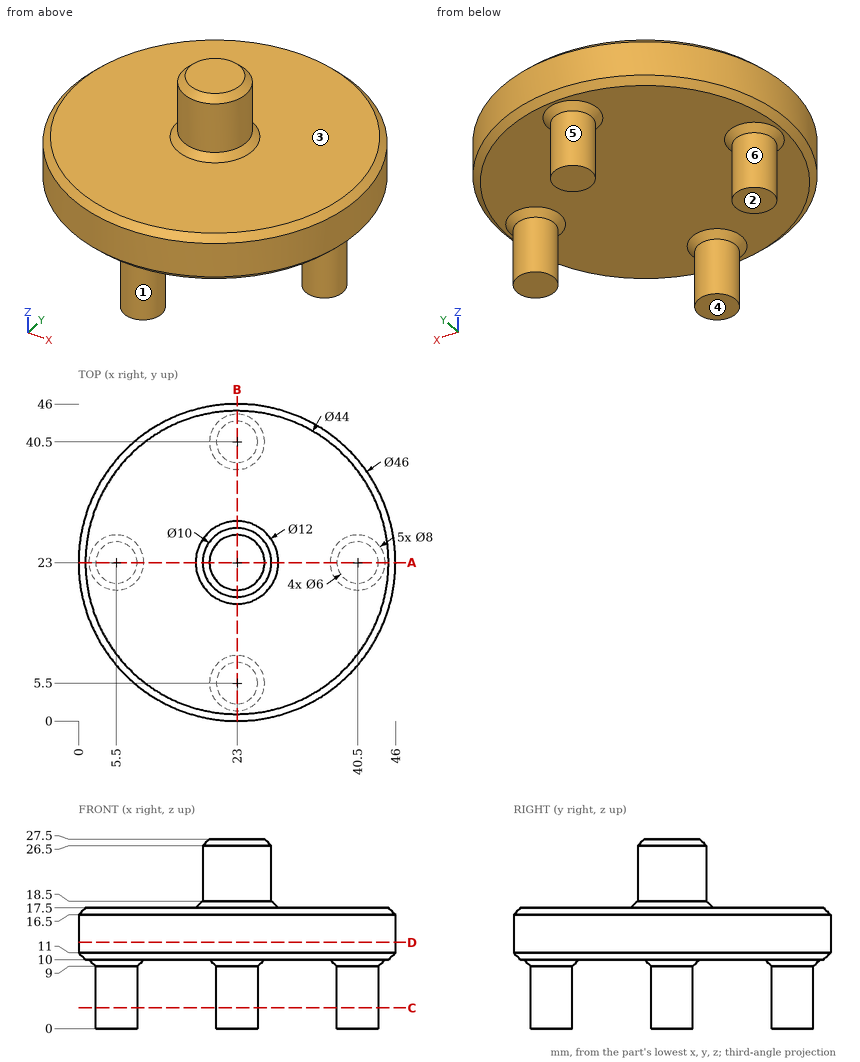
For this review, use the dimensioned drawing (mm, ordinates from the lowest corner) and the shaded views. A direction names the side the tool comes from. Give positions to 0.01 mm unless a question says otherwise; leave off trailing zeros. Write each loop counter-clockwise with the first axis right and the second up, starting at its lowest first coordinate (ties: lowest second). Pieces come first, ordered by that corner, then holes.
(1) Consider section A-A, the plane y = 23. Give the boundary of the cut face in (x, z).
(2) The part is to be moulded in two halves that separate along X. For the marked faces 4, 5 and 6, say which applies: released by +X, released by -X, zero draft, split by the parting line, or undercut.
(3) Consider section D-D, the plane z = 12.5. Give the boundary of the cut face in (x, y).
(4) For P1, Ø6, axis at y = 40.5, z = 14.5, coming from the +X side; P2, Ø10, axis at x = 20.5, z = 17, coming from the -Y side; P3, Ø10, axis at x = 15.5, y = 13, coming from the -Z side, all flat-tipped, find the tip position at first contact; note any pin that passes through.
(5) Consider section C-C, the plane z = 3. Give the boundary of the cut face in (x, y).
(6) Tool access review of the marked faces 1, 2 and 3: name each direction out of +Z, -Z, +X, -X, +Y, -Y from which nothing blocks a thin tool from reaching the whole face with its end or side.
(7) To check wall thickness, follow L1, parallel to Z at x = 13, y = 22.5; L2, parallel to Z at x = 4.5, y = 22.5; L3, parallel to Y at x = 2, z = 12. State the ranges of each line that lie inside material, in increasing order.
Returned:
1. outline: (0, 11) - (1, 10) - (1.5, 10) - (2.5, 9) - (2.5, 0) - (8.5, 0) - (8.5, 9) - (9.5, 10) - (36.5, 10) - (37.5, 9) - (37.5, 0) - (43.5, 0) - (43.5, 9) - (44.5, 10) - (45, 10) - (46, 11) - (46, 16.5) - (45, 17.5) - (29, 17.5) - (28, 18.5) - (28, 26.5) - (27, 27.5) - (19, 27.5) - (18, 26.5) - (18, 18.5) - (17, 17.5) - (1, 17.5) - (0, 16.5) - close
2. face 4: zero draft
2. face 5: split by the parting line
2. face 6: undercut
3. outline: circle Ø46 at (23, 23)
4. P1: stops at x = 40.85
4. P2: stops at y = 0
4. P3: stops at z = 10
5. outline: circle Ø6 at (5.5, 23); circle Ø6 at (23, 5.5); circle Ø6 at (23, 40.5); circle Ø6 at (40.5, 23)
6. face 1: -Z
6. face 2: -Z, +X, -X, +Y, -Y
6. face 3: +Z
7. L1: z = 10 to 17.5
7. L2: z = 0 to 17.5
7. L3: y = 13.62 to 32.38
